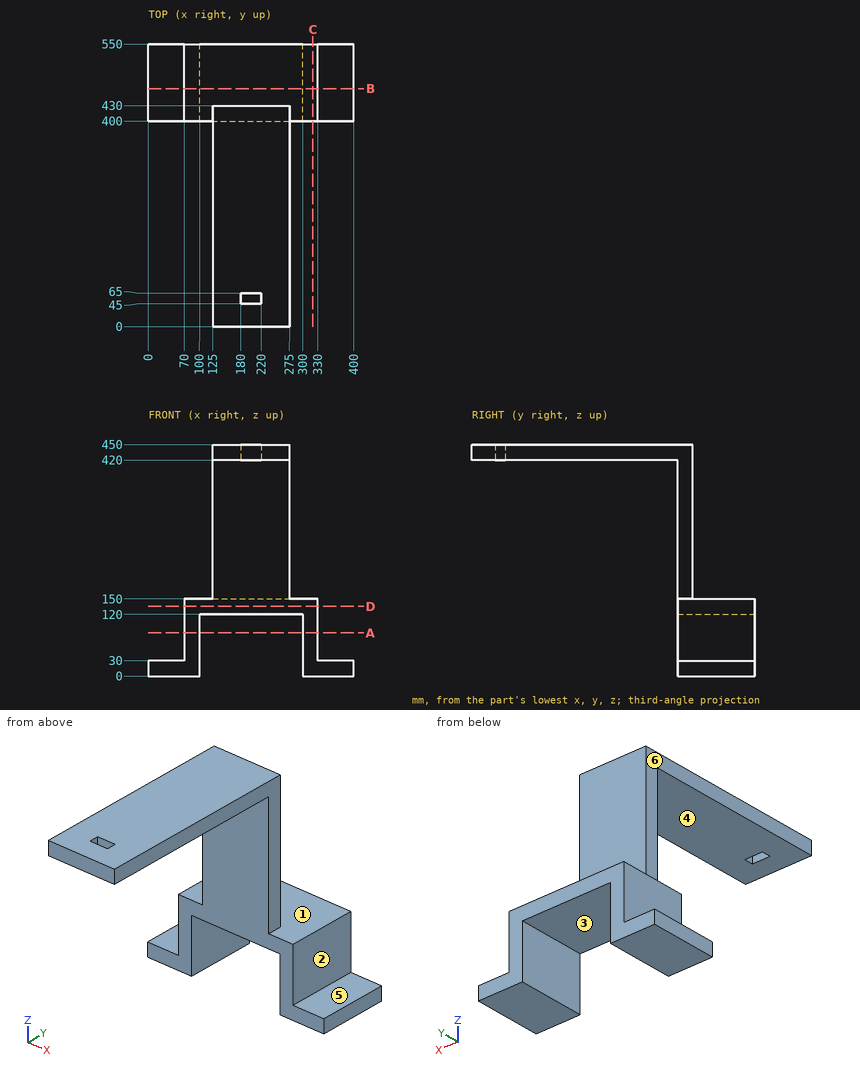
Part print with two shaded views. Sizes in mm from the minimum x, y, z corner. A direction names the side the tool comes from. Round coordinates to 2 decimals unless told otherwise and drop trailing zeros. Loops run counter-clockwise (first coordinate to the right, second up) from the corner with the lowest first, then second, coordinate; pieces in that order, holes last. Notation, with made-up numbers: M 48.25,39.5 L 81.25,39.5 A29 ccw 81.25,72.5 Z; hole C 30.25,66 d3. An arc over 180 degrees is marked long. Return JSON: item names as keys, results as strings. Group by question number.
(1) Saw through at B-B, the plane y = 463. List the corners of the cut face in (x, z), and give its area (3 significant figures).
(2) Saw through at A-A, the plane z = 84. List the corners of the cut face in (x, y), and give its area (3 significant figures).
(3) Wall check: probe 1 along Z at (x, y) = (21, 470); probe 2 along X at (y, z) = (52, 425.5); probe 3 along Y at (x, z) = (250, 220.5). Give the ranges that are in metal, low to high. Write a range as [from, to].
(4) Mould opens along X. For the marked faces 1, 2 and 3 say: +X half, -X half, draft (parallel to the pull), parting line (faces both ways), or undercut.
(5) Drop flat-ended pins along their axis: P1, Ø10, axis at y = 52.5, z = 428.5, coming from the +X side; P2, Ø1, axis at x = 156.5, z = 316, coming from the +Y side; P3, Ø1.5, axis at y = 446.5, z = 74, coming from the +X side. Give the stop position or say it passes through.
(6) Saw through at D-D, the plane z = 135.5. List the corners of the cut face in (x, y), and give its area (3 significant figures).
(7) Saw through at C-C, the plane x = 320. List the corners of the cut face in (y, z).
(8) Tool access for the marked faces 4, 5 and 6: list every direction of +Z, -Z, +X, -X, +Y, -Y with a clear straight run to the whole face (end or side of a thin tool).
Answer list:
{
 "1": {"outline": "M 0,0 L 100,0 L 100,120 L 300,120 L 300,0 L 400,0 L 400,30 L 330,30 L 330,150 L 70,150 L 70,30 L 0,30 Z", "area": "19,200 mm2"},
 "2": {"outline": "M 70,400 L 100,400 L 100,550 L 70,550 Z; M 300,400 L 330,400 L 330,550 L 300,550 Z", "area": "9,000 mm2"},
 "3": {"probe 1": "[0, 30]", "probe 2": "[125, 180], [220, 275]", "probe 3": "[400, 430]"},
 "4": {"face 1": "draft", "face 2": "+X half", "face 3": "undercut"},
 "5": {"P1": "x = 275", "P2": "y = 430", "P3": "x = 330"},
 "6": {"outline": "M 70,400 L 330,400 L 330,550 L 70,550 Z", "area": "39,000 mm2"},
 "7": {"outline": "M 400,0 L 550,0 L 550,150 L 400,150 Z"},
 "8": {"face 4": "-Z, +X, -X, -Y", "face 5": "+Z, +X, +Y, -Y", "face 6": "+Z, -X, +Y, -Y"}
}
